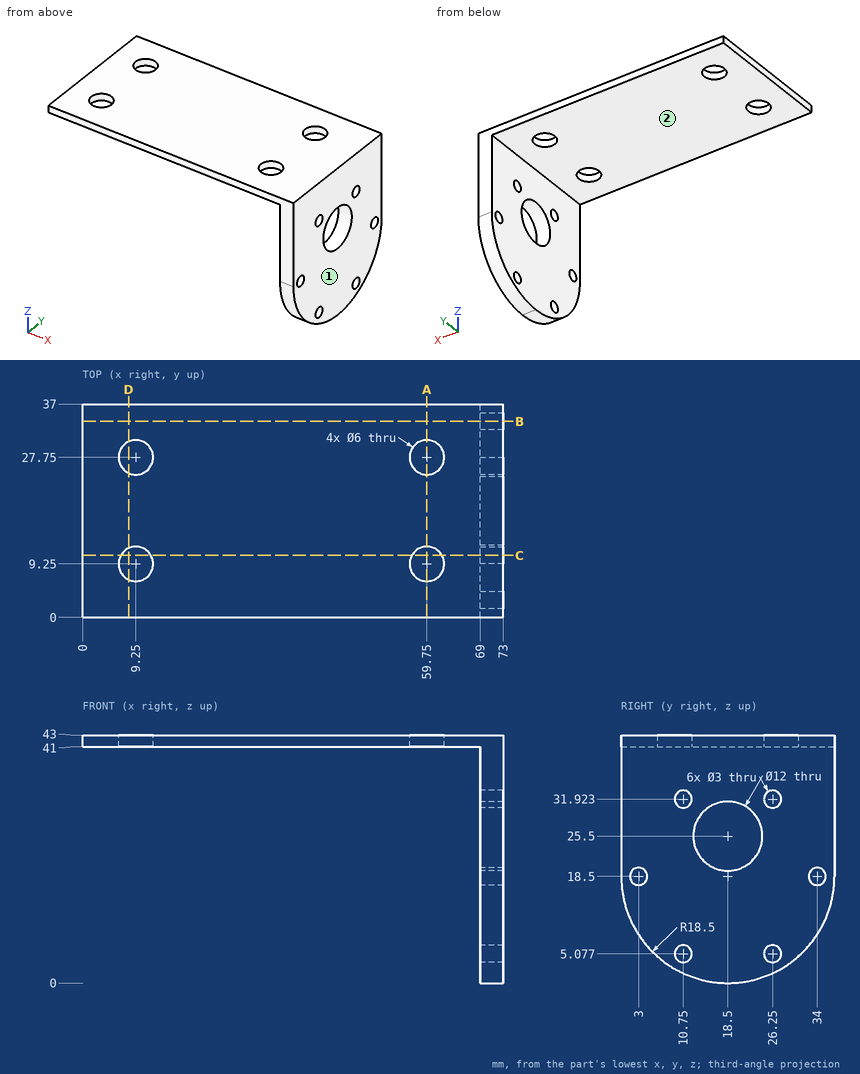
For this review, use the dimensioned drawing (mm, ordinates from the lowest corner) and the shaded views. A direction names the side the tool comes from. Give positions to 0.01 mm unless a question says otherwise; leave off trailing zeros. Write each loop counter-clockwise with the first axis right and the second up, starting at its lowest first coordinate (ties: lowest second). Pieces come first, ordered by that corner, then holes.
(1) For P1, Ø7, axis at x = 59.75, y = 9.25, coming from the +Z side; P2, Ø2.5, axis at y = 26.25, z = 31.92, coming from the +X side; P3, Ø8, axis at x = 59.75, y = 27.75, coming from the -Z side; P4, Ø15.5, axis at y = 18.5, z = 25.5, coming from the -X side, all flat-tipped, find the tip position at first contact; note any pin that passes through.
(2) Consider section A-A, the plane x = 59.75. Give the boundary of the cut face in (y, z), and give its area (3 significant figures).
(3) Consider section D-D, the plane x = 8. Give the boundary of the cut face in (y, z).
(4) Consider section B-B, the plane y = 34. Give the boundary of the cut face in (x, z).
(5) Consider section C-C, the plane y = 10.75. Give the boundary of the cut face in (x, z).
(6) To check wall thickness, follow L1, parallel to Y at x = 9.25, z = 41.45; L2, parallel to Y at x = 70, z = 18 (1 decimal); L3, parallel to Z at x = 71, y = 26 (1 decimal). State the ranges of each line that lie inside material, in increasing order.
(7) Tool access review of the marked faces 1 and 2: name each direction out of +Z, -Z, +X, -X, +Y, -Y from which nothing blocks a thin tool from reaching the whole face with its end or side.
Returned:
1. P1: stops at z = 43
1. P2: passes through
1. P3: stops at z = 41
1. P4: stops at x = 69
2. outline: (0, 41) - (6.25, 41) - (6.25, 43) - (0, 43) - close; (12.25, 41) - (24.75, 41) - (24.75, 43) - (12.25, 43) - close; (30.75, 41) - (37, 41) - (37, 43) - (30.75, 43) - close
2. area: 50.0 mm2
3. outline: (0, 41) - (6.52, 41) - (6.52, 43) - (0, 43) - close; (11.98, 41) - (25.02, 41) - (25.02, 43) - (11.98, 43) - close; (30.48, 41) - (37, 41) - (37, 43) - (30.48, 43) - close
4. outline: (0, 41) - (69, 41) - (69, 20) - (73, 20) - (73, 43) - (0, 43) - close; (69, 8.4) - (73, 8.4) - (73, 17) - (69, 17) - close
5. outline: (0, 41) - (6.65, 41) - (6.65, 43) - (0, 43) - close; (11.85, 41) - (57.15, 41) - (57.15, 43) - (11.85, 43) - close; (62.35, 41) - (69, 41) - (69, 33.42) - (73, 33.42) - (73, 43) - (62.35, 43) - close; (69, 1.7) - (73, 1.7) - (73, 3.58) - (69, 3.58) - close; (69, 6.58) - (73, 6.58) - (73, 30.42) - (69, 30.42) - close
6. L1: y = 0 to 6.25, 12.25 to 24.75, 30.75 to 37
6. L2: y = 0 to 1.6, 4.4 to 32.6, 35.4 to 37
6. L3: z = 1.6 to 3.6, 6.6 to 30.4, 33.4 to 43
7. face 1: +Z, -Z, +X, +Y, -Y
7. face 2: -Z, -X, +Y, -Y
